Autodesk Inventor part; units mm, degrees
ref_plane "YZ Plane" through (0, 0, 0) normal (1, 0, 0) x (0, 1, 0)
ref_plane "XZ Plane" through (0, 0, 0) normal (0, 1, 0) x (-1, 0, 0)
ref_plane "XY Plane" through (0, 0, 0) normal (0, 0, 1) x (1, 0, 0)
sketch "Sketch1" plane through (0, 0, 0) normal (0, 0, 1) x (1, 0, 0)
  circle A0 centre (0, 0) radius 28
  circle A1 centre (0, 0) radius 17
  point P0 (0, 22)
  dimension "d0" = 22
  dimension "d1" = 34
  dimension "d20" = 56
extrude "Extrusion1" add sketch "Sketch1" along normal mid plane 8
sketch "Sketch2" plane through (0, 0, 4) normal (0, 0, 1) x (1, 0, 0)
  point P0 (0, 0)
  point P1 (0, 22)
  dimension "d4" = 22
hole "Hole1" at (0, 22, 4) direction (0, 0, -1) diameter 5 end through all
pattern_circular "Circular Pattern1" count 6 over 360 about axis through (0, 0, -10) along (0, 0, 1) of "Hole1"
sketch "Sketch3" plane through (0, 0, 4) normal (0, 0, 1) x (1, 0, 0)
  circle A0 centre (0, 22) radius 2.5
  circle A1 centre (19.0526, 11) radius 2.5
  line L0 (0, 22) -> (19.0526, 11) construction
  circle A2 centre (17.4522, 30.2282) radius 12.7296
  line L1 (9.5263, 16.5) -> (19.9795, 34.6056) construction
  point P0 (0, 0)
extrude "Extrusion2" cut sketch "Sketch3" against normal blind 8 contours A2
pattern_circular "Circular Pattern2" count 6 over 360 about axis through (0, 0, -10) along (0, 0, 1) of "Extrusion2"
properties part number "Spacer8mm"
Model file for the job. Use its own axes, mm. Coordinates: 2 decimals unless noted, no trailing zeros. Write each loop counter-clockwise with the first axis right and the second up, starting at its lowest first coordinate (ties: lowest second). Pieces come first, ordered by that corner, then holes. Notation, with made-up numbers: (46, -36) - (57, -36) arc R23 cw to (57, -1) - close; hole circle Ø3 at (-21, -18). An arc over 180 degrees is marked (long way). One line per item, written item: value. Start each with the question number.
1. Slice it at C-C (x = -6.5). Write the cut outline in (y, z), plus the area to 3 significant figures.
2. Probe line 1 (X direction, y = 11, z = 1); line 2 (X direction, y = -10.5, z = 3.5); line 3 (Y direction, x = 20.5, z = 2.25). List the from-to ranges inside material, lowest first. Write a range as from..to.
3. Flat gauge pins, fed straight in: pin 1 (2 mm diameter, centred on x = -20.5, z = -0.5, fed in from +Y); pin 2 (3 mm diameter, centred on x = 19.05, y = 11, fed in from -Z); pin 3 (1 mm diameter, centred on y = -17.5, z = 0.5, fed in from -X); pin 4 (3 mm diameter, centred on y = -18, z = 1, fed in from -X). Where does each tip first touch, or does it go through?
4. Slice it at A-A (x = 0). Write the cut outline in (y, z).
5. Slice it at B-B (y = 0). Write the cut outline in (x, z).
6. Mould opens along Y. For faces 1 (the cylindrical face through (10.96, 19.28, 0.06)), 2 (the cylindrical face through (22.176, 0.149, 0.056)), 3 (the cylindrical face through (11.22, -19.13, 0.06)) say: released by +Y, released by -Y, zero draft, split by the parting line, or undercut.
7. Slice it at D-D (z = 2). Write the cut outline in (x, y), plus the area to 3 significant figures.
Answers below:
1. outline: (-23.74, -4) - (-15.71, -4) - (-15.71, 4) - (-23.74, 4) - close; (15.71, -4) - (23.74, -4) - (23.74, 4) - (15.71, 4) - close
1. area: 129 mm^2
2. line 1: x = -25.75..-21.55, -16.55..-12.96, 12.96..16.55, 21.55..25.75
2. line 2: x = -25.96..-21.5, -16.6..-13.37, 13.37..16.6, 21.5..25.96
2. line 3: y = -17.87..-13.04, -8.96..8.96, 13.04..17.87
3. pin 1: stops at y = 18.11
3. pin 2: passes through
3. pin 3: stops at x = -22.25
3. pin 4: stops at x = -22.62
4. outline: (-28, -4) - (-24.5, -4) - (-24.5, 4) - (-28, 4) - close; (-19.5, -4) - (-17, -4) - (-17, 4) - (-19.5, 4) - close; (17, -4) - (19.5, -4) - (19.5, 4) - (17, 4) - close; (24.5, -4) - (28, -4) - (28, 4) - (24.5, 4) - close
5. outline: (-22.17, -4) - (-17, -4) - (-17, 4) - (-22.17, 4) - close; (17, -4) - (22.17, -4) - (22.17, 4) - (17, 4) - close
6. face 1: released by +Y
6. face 2: undercut
6. face 3: released by -Y
7. outline: (-26.36, -9.44) arc R28 ccw to (-21.35, -18.11) arc R12.73 cw to (-5.01, -27.55) arc R28 ccw to (5.01, -27.55) arc R12.73 cw to (21.35, -18.11) arc R28 ccw to (26.36, -9.44) arc R12.73 cw to (26.36, 9.44) arc R28 ccw to (21.35, 18.11) arc R12.73 cw to (5.01, 27.55) arc R28 ccw to (-5.01, 27.55) arc R12.73 cw to (-21.35, 18.11) arc R28 ccw to (-26.36, 9.44) arc R12.73 cw to start; hole circle Ø5 at (-19.05, -11); hole circle Ø5 at (-19.05, 11); hole circle Ø34 at (0, 0); hole circle Ø5 at (0, -22); hole circle Ø5 at (0, 22); hole circle Ø5 at (19.05, -11); hole circle Ø5 at (19.05, 11)
7. area: 985 mm^2
